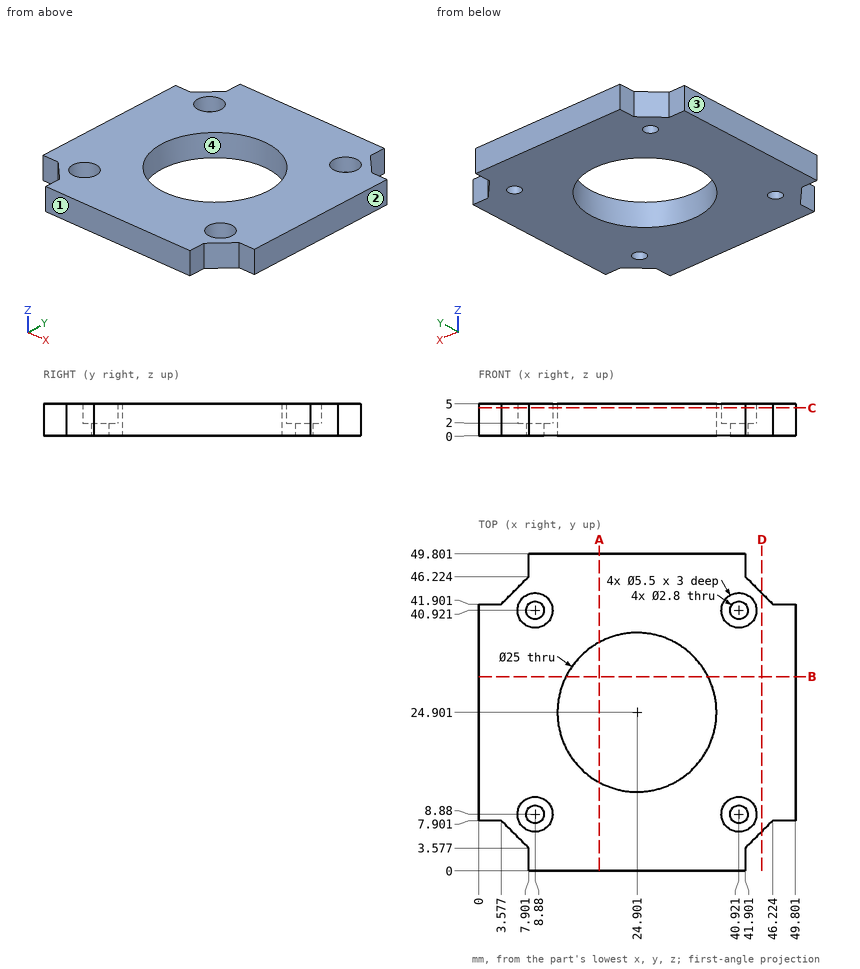
Drawing for the job (mm, zero at the part's lowest x, y, z). Round coordinates to 2 decimals unless told otherwise and drop trailing zeros. Loops run counter-clockwise (first coordinate to the right, second up) from the corner with the lowest first, then second, coordinate; pieces in that order, holes last. Notation, with made-up numbers: M -6,75 L 5,75 A26 cw 5,108 Z; hole C 3,84.25 d7. An arc over 180 degrees is marked long. Use a Markdown table: item, result. Add a question column.
(1) Cut at C-C (z = 4.4). Give the cut face in (x, y), and give its area (3 significant figures).
(2) Drill centre lines: line 1 (Y direction, x = 9, z = 4.1); line 2 (X direction, y = 41, z = 0.45). Where is each one in solid material? Low to high.
(3) Cut at D-D (x = 44.5). Give the cut face in (y, z) (1 decimal), and give its area (3 significant figures).
(4) Flat gauge pins, fed straight in: pin 1 (1.1 mm diameter, centred on y = 48.5, z = 2.5, fed in from -X); pin 2 (1.6 mm diameter, centred on x = 9.5, y = 41.5, fed in from +Z); pin 3 (3 mm diameter, centred on x = 2, z = 2.5, fed in from +Y). Where does each tip first touch, or does it go through?
(5) Cut at B-B (y = 30.5). Give the cut face in (x, z) (1 decimal), and give its area (3 significant figures).
(6) Cut at A-A (x = 19). Give the cut face in (y, z).
(7) Pull direction X, two halves, no side cores. Call the marked faces 1, 2, 3 and 4: +X half, -X half, draft (parallel to the pull), parting line (faces both ways), or undercut.
Geometry says:
| question | item | result |
|---|---|---|
| 1 | outline | M 0,7.9 L 3.58,7.9 L 7.9,3.58 L 7.9,0 L 41.9,0 L 41.9,3.58 L 46.22,7.9 L 49.8,7.9 L 49.8,41.9 L 46.22,41.9 L 41.9,46.22 L 41.9,49.8 L 7.9,49.8 L 7.9,46.22 L 3.58,41.9 L 0,41.9 Z; hole C 8.88,8.88 d5.5; hole C 8.88,40.92 d5.5; hole C 24.9,24.9 d25; hole C 40.92,8.88 d5.5; hole C 40.92,40.92 d5.5 |
| 1 | area | 1,680 mm² |
| 2 | line 1 | y = 0 to 6.13, 11.63 to 38.17, 43.67 to 49.8 |
| 2 | line 2 | x = 0 to 7.48, 10.28 to 39.52, 42.32 to 49.8 |
| 3 | outline | M 6.2,0 L 43.6,0 L 43.6,5 L 6.2,5 Z |
| 3 | area | 187 mm² |
| 4 | pin 1 | stops at x = 7.9 |
| 4 | pin 2 | stops at z = 2 |
| 4 | pin 3 | stops at y = 41.9 |
| 5 | outline | M 0,0 L 13.7,0 L 13.7,5 L 0,5 Z; M 36.1,0 L 49.8,0 L 49.8,5 L 36.1,5 Z |
| 5 | area | 137 mm² |
| 6 | outline | M 0,0 L 13.88,0 L 13.88,5 L 0,5 Z; M 35.92,0 L 49.8,0 L 49.8,5 L 35.92,5 Z |
| 7 | face 1 | draft |
| 7 | face 2 | +X half |
| 7 | face 3 | -X half |
| 7 | face 4 | undercut |
